Could you check a few things on this model? Use its own coordinates, in mm. A direction names the side the tool comes from. Give positions to 0.01 mm unless a question says otherwise; leave off trailing zeros. Order: outer loops, then holes, each group sorted by start corner. A loop starts at its lowest first (then second) coordinate and runs counter-clockwise, first axis right, second up.
(1) Imagine slicing it at C-C, the plane x = 0. Write out the boundary of the cut face in (y, z), then the cut area to 3 significant figures.
(2) Imagine slicing it at B-B, the plane z = 50.8. Write out the boundary of the cut face in (x, y), then the cut area to 3 significant figures.
(3) If we mould it in two halves opening along X, with no side actions, what happens to faces 1 (the flat face through (-48, 3, 63.5)), 2 (the cylindrical face through (-51.9, 3.13, -47.32)), 3 (the flat face through (63.5, 3, -1))? For each: released by +X, released by -X, zero draft, split by the parting line, or undercut.
(4) On a 3-axis mill with a long thin cutter (end or side, diameter ignored), from which of +Z, -Z, +X, -X, +Y, -Y can I reach the whole of each face in a straight line? I mean faces 4 (the flat face through (48, 3, 63.5)), 5 (the flat face through (-32.5, 3, 49)). Say none if no direction works.
(5) Imagine slicing it at A-A, the plane x = -50.8. Write out the boundary of the cut face in (y, z), then the cut area to 3 significant figures.
(6) If I drill on probe 1 along Z at (x, y) = (0, 4.5); probe 2 along X at (y, z) = (2.5, 0); probe 3 along X at (y, z) = (4, -25.4), over which ranges is the centre line in solid material (lowest first)?
(7) Will this pin go through, and if not, where does the flat tip stop? pin 1 (2 mm diameter, centred on x = -27, y = 5.5, fed in from +Z).
(8) Imagine slicing it at D-D, the plane y = 4.25. State how many separate pieces and enclosed holes the cut face has, then the cut area to 3 significant figures.
Autodesk Inventor part; units mm, degrees
ref_plane "YZ Plane" through (0, 0, 0) normal (1, 0, 0) x (0, 1, 0)
ref_plane "XZ Plane" through (0, 0, 0) normal (0, 1, 0) x (-1, 0, 0)
ref_plane "XY Plane" through (0, 0, 0) normal (0, 0, 1) x (1, 0, 0)
sketch "Sketch3" plane through (0, 0, 0) normal (0, 1, 0) x (-1, 0, 0)
  circle A0 centre (0, 29.3624) radius 3.6195
  circle A1 centre (0, 29.3624) radius 3.6195
  circle A2 centre (25.4286, 14.6812) radius 3.6195
  circle A3 centre (-25.4286, 14.6812) radius 3.6195
  circle A4 centre (-25.4286, -14.6812) radius 3.6195
  circle A5 centre (0, -29.3624) radius 3.6195
  circle A6 centre (25.4286, -14.6812) radius 3.6195
  circle A7 centre (-25.4286, 14.6812) radius 3.6195
  circle A8 centre (-25.4286, -14.6812) radius 3.6195
  circle A9 centre (0, -29.3624) radius 3.6195
  circle A10 centre (25.4286, -14.6812) radius 3.6195
  circle A11 centre (25.4286, 14.6812) radius 3.6195
  line L0 (-63.5, 63.5) -> (63.5, 63.5)
  line L1 (63.5, 63.5) -> (63.5, -63.5)
  line L2 (63.5, -63.5) -> (-63.5, -63.5)
  line L3 (-63.5, -63.5) -> (-63.5, 63.5)
  line L4 (-63.5, 63.5) -> (63.5, -63.5) construction
  line L5 (63.5, 63.5) -> (-63.5, -63.5) construction
  point P0 (0, 0)
  dimension "d104" = 127
  dimension "d105" = 127
extrude "Extrusion1" add sketch "Sketch3" along normal blind 6.35
sketch "Sketch4" plane through (0, 0, 0) normal (0, -1, 0) x (1, 0, 0)
  circle A0 centre (-50.8, -50.8) radius 3
  line L0 (-63.5, -63.5) -> (-63.5, 63.5)
  line L1 (63.5, -63.5) -> (-63.5, -63.5)
  circle A1 centre (50.8, -50.8) radius 3
  line L2 (63.5, 63.5) -> (63.5, -63.5)
  circle A2 centre (50.8, 50.8) radius 3
  line L3 (-63.5, 63.5) -> (63.5, 63.5)
  circle A3 centre (-50.8, 50.8) radius 3
  point P0 (0, 0)
  dimension "d106" = 6
  dimension "d107" = 12.7
  dimension "d108" = 12.7
  dimension "d109" = 6
  dimension "d110" = 12.7
  dimension "d111" = 12.7
  dimension "d112" = 6
  dimension "d113" = 12.7
  dimension "d114" = 12.7
  dimension "d115" = 6
  dimension "d116" = 12.7
  dimension "d117" = 12.7
hole "Hole6" at (-50.8, 0, 50.8) direction (0, 1, 0) diameter 6 end through all
hole "Hole7" at (50.8, 0, 50.8) direction (0, 1, 0) diameter 6 end through all
hole "Hole8" at (50.8, 0, -50.8) direction (0, 1, 0) diameter 6 end through all
hole "Hole9" at (-50.8, 0, -50.8) direction (0, 1, 0) diameter 6 end through all
hole "Hole10" at (0, 0, 0) direction (0, 1, 0) diameter 38.1 end through all
pattern_linear "Rectangular Pattern5" count 4 spacing 25.4 along (0, 0, -1) of "Hole6"
pattern_linear "Rectangular Pattern6" count 4 spacing 25.4 along (1, 0, 0) of "Hole6"
pattern_linear "Rectangular Pattern7" count 4 spacing 25.4 along (0, 0, -1) of "Hole7"
pattern_linear "Rectangular Pattern8" count 4 spacing 25.4 along (-1, 0, 0) of "Hole8"
thread "Thread21"
thread "Thread22"
thread "Thread23"
thread "Thread24"
thread "Thread25"
thread "Thread26"
thread "Thread27"
thread "Thread28"
thread "Thread29"
thread "Thread30"
thread "Thread31"
thread "Thread32"
sketch "Sketch6" plane through (0, 6.35, 0) normal (0, 1, 0) x (1, 0, 0)
  line L0 (-32.5, -92.5) -> (32.5, -92.5)
  line L1 (32.5, -92.5) -> (32.5, -34.5)
  line L2 (32.5, -34.5) -> (-32.5, -34.5)
  line L3 (-32.5, -34.5) -> (-32.5, -92.5)
  line L4 (-63.5, -63.5) -> (63.5, -63.5)
  line L5 (-32.5, -92.5) -> (32.5, -34.5) construction
  line L6 (32.5, -92.5) -> (-32.5, -34.5) construction
  point P0 (0, 0)
  point P1 (0, -63.5)
  dimension "d189" = 65
  dimension "d232" = 58
extrude "Extrusion2" cut sketch "Sketch6" against normal blind 25.4
sketch "Sketch7" plane through (0, 6.35, 0) normal (0, 1, 0) x (1, 0, 0)
  circle A0 centre (-50.8, -50.8) radius 3
  line L0 (-63.5, -63.5) -> (-63.5, 63.5)
  line L1 (63.5, -63.5) -> (-63.5, -63.5)
  circle A1 centre (50.8, -50.8) radius 3
  line L2 (63.5, 63.5) -> (63.5, -63.5)
  circle A2 centre (50.8, 50.8) radius 3
  line L3 (-63.5, 63.5) -> (63.5, 63.5)
  circle A3 centre (-50.8, 50.8) radius 3
  point P0 (0, 0)
  point P1 (0, 0)
  dimension "d192" = 6
  dimension "d193" = 12.7
  dimension "d194" = 12.7
  dimension "d195" = 6
  dimension "d196" = 12.7
  dimension "d197" = 12.7
  dimension "d198" = 6
  dimension "d199" = 12.7
  dimension "d200" = 12.7
  dimension "d201" = 6
  dimension "d202" = 12.7
  dimension "d203" = 12.7
hole "Hole11" at (-50.8, 6.35, -50.8) direction (0, -1, 0) diameter 7.3 end through all
hole "Hole12" at (50.8, 6.35, -50.8) direction (0, -1, 0) diameter 7.3 end through all
hole "Hole13" at (50.8, 6.35, 50.8) direction (0, -1, 0) diameter 7.3 end through all
hole "Hole14" at (-50.8, 6.35, 50.8) direction (0, -1, 0) diameter 7.3 end through all
properties part number "basenueva(5x5)"
Answer block:
1. outline: (0, -63.5) - (6.35, -63.5) - (6.35, -53.8) - (0, -53.8) - close; (0, -47.8) - (6.35, -47.8) - (6.35, -32.98) - (0, -32.98) - close; (0, -25.74) - (6.35, -25.74) - (6.35, -19.05) - (0, -19.05) - close; (0, 19.05) - (6.35, 19.05) - (6.35, 25.74) - (0, 25.74) - close; (0, 32.98) - (6.35, 32.98) - (6.35, 34.5) - (0, 34.5) - close
1. area: 250 mm2
2. outline: (-63.5, 0) - (-54.45, 0) - (-54.45, 6.35) - (-63.5, 6.35) - close; (-47.15, 0) - (-32.5, 0) - (-32.5, 6.35) - (-47.15, 6.35) - close; (32.5, 0) - (47.15, 0) - (47.15, 6.35) - (32.5, 6.35) - close; (54.45, 0) - (63.5, 0) - (63.5, 6.35) - (54.45, 6.35) - close
2. area: 301 mm2
3. face 1: zero draft
3. face 2: undercut
3. face 3: released by +X
4. face 4: +Z, +X, -X, +Y, -Y
4. face 5: +Z, +Y, -Y
5. outline: (0, -63.5) - (6.35, -63.5) - (6.35, -54.45) - (0, -54.45) - close; (0, -47.15) - (6.35, -47.15) - (6.35, -28.4) - (0, -28.4) - close; (0, -22.4) - (6.35, -22.4) - (6.35, -3) - (0, -3) - close; (0, 3) - (6.35, 3) - (6.35, 22.4) - (0, 22.4) - close; (0, 28.4) - (6.35, 28.4) - (6.35, 47.15) - (0, 47.15) - close; (0, 54.45) - (6.35, 54.45) - (6.35, 63.5) - (0, 63.5) - close
5. area: 599 mm2
6. probe 1: z = -63.5 to -53.8, -47.8 to -32.98, -25.74 to -19.05, 19.05 to 25.74, 32.98 to 34.5
6. probe 2: x = -63.5 to -53.8, -47.8 to -19.05, 19.05 to 47.8, 53.8 to 63.5
6. probe 3: x = -63.5 to -53.8, -47.8 to 47.8, 53.8 to 63.5
7. pin 1: stops at z = 34.5
8. separate pieces: 1
8. enclosed holes: 20
8. area: 12,400 mm2
